Here's the drawing with two shaded views (mm, measured from the low corner). I have some questions. A direction names the side the tool comes from. Coordinates: 2 decimals unless noted, no trailing zeros. Order: outer loops, then holes, each group sorted by start corner. A loop starts at its lowest first (then second) coordinate and runs counter-clockwise, first axis right, second up. Notation, with made-up numbers: (-8.75, 79) -> (33.25, 79) arc R19 cw to (33.25, 114) -> close; hole circle Ø1 at (86.5, 59.25). An arc over 180 degrees is marked (long way). Answer as a JSON object with one key per item and string values. Group by question number.
(1) For pin 1 (1 mm diameter, centred on x = 3.5, y = 7.5, fed in from -Z); pin 2 (2 mm diameter, centred on x = 2, y = 8, fed in from +Z); pin 3 (1.5 mm diameter, centred on y = 1.5, z = 2.5, fed in from -X), each with a flat end and sliding along its axis, tell me the tip position at first contact or that it passes through.
(2) I need wall thicknesses on line 1 (Y direction, x = 1.7, z = 1.3); line 2 (Y direction, x = 3.6, z = 2.5); line 3 (Z direction, x = 2.6, y = 8.5). Which ranges of each line are inside material? Lowest first, please.
(3) If we mould it in two halves opening along Z, with no side actions, what happens to the marked faces 3 and 4? For each: pulls with the +Z half, pulls with the -Z half, needs draft (parallel to the pull), parting line crosses it, or undercut.
(4) I want a section at A-A, the plane z = 1.9. List the corners of the cut face in (x, y) for me.
(5) I want a section at C-C, the plane y = 1. List the corners of the cut face in (x, z) for me.
(6) Which directions (+Z, -Z, +X, -X, +Y, -Y) give clear straight access to the entire face, cutting with the end or side of a thin tool? Please do the marked faces 1 and 2.
(7) I want a section at D-D, the plane y = 6.75. List the corners of the cut face in (x, z) for me.
(8) I want a section at B-B, the plane x = 1.9. List the corners of the cut face in (y, z) for me.
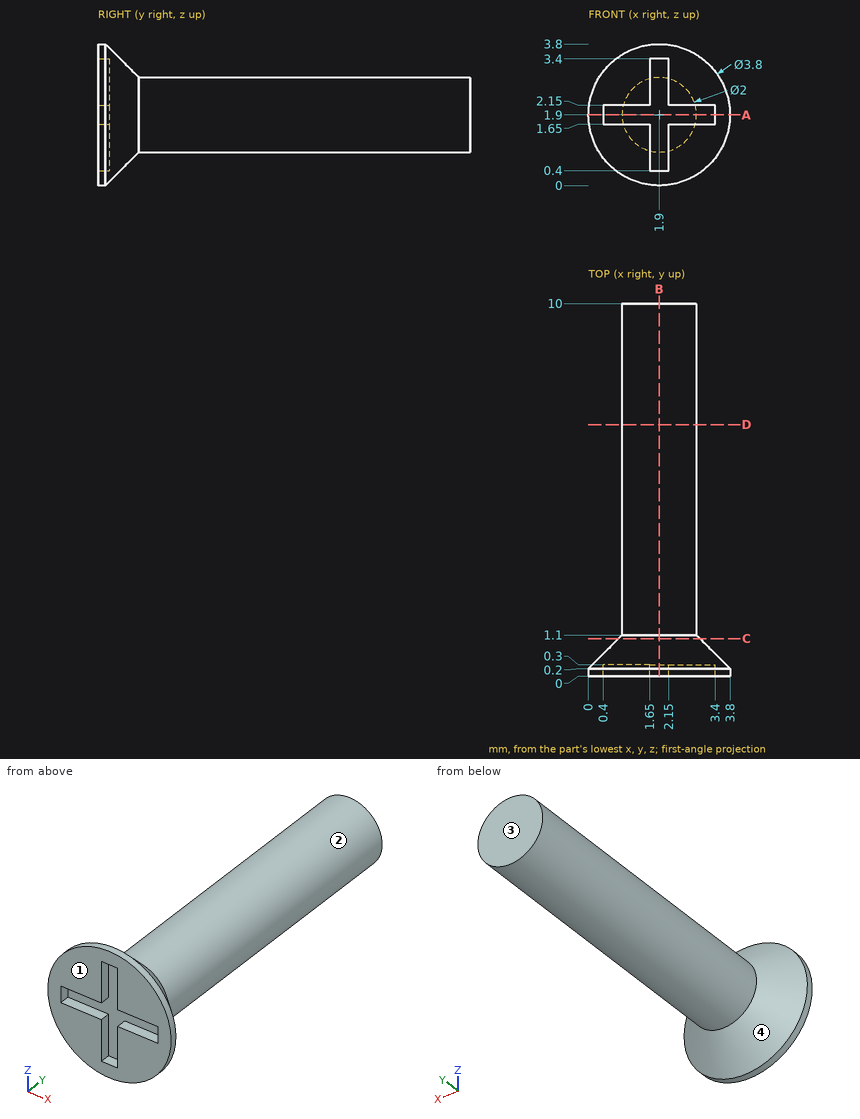
Computed values:
{
 "1": {"pin 1": "passes through", "pin 2": "stops at z = 2.9", "pin 3": "stops at x = 0.64"},
 "2": {"line 1": "y = 0.3 to 10", "line 2": "y = 0 to 0.3", "line 3": "z = 1.19 to 2.61"},
 "3": {"face 3": "needs draft", "face 4": "parting line crosses it"},
 "4": {"outline": "(0, 0) -> (0.4, 0) -> (0.4, 0.3) -> (3.4, 0.3) -> (3.4, 0) -> (3.8, 0) -> (3.8, 0.2) -> (2.9, 1.1) -> (2.9, 10) -> (0.9, 10) -> (0.9, 1.1) -> (0, 0.2) -> close"},
 "5": {"outline": "circle Ø2.2 at (1.9, 1.9)"},
 "6": {"face 1": "+Z, -Z, +X, -X, -Y", "face 2": "+Y"},
 "7": {"outline": "circle Ø2 at (1.9, 1.9)"},
 "8": {"outline": "(0, 0) -> (0.2, 0) -> (1.1, 0.9) -> (10, 0.9) -> (10, 2.9) -> (1.1, 2.9) -> (0.2, 3.8) -> (0, 3.8) -> (0, 3.4) -> (0.3, 3.4) -> (0.3, 0.4) -> (0, 0.4) -> close"}
}
